Geometry check sheet. Reference: the model listing, model coordinates, mm. A direction names the side the tool comes from. Round coordinates to 2 decimals unless told otherwise and drop trailing zeros. Order: outer loops, then holes, each group sorted by start corner. A loop starts at its lowest first (then second) coordinate and runs counter-clockwise, first axis right, second up.
```python
from build123d import *

# Parameters (mm, degrees)
ESQUISSE1_W     = 40
ESQUISSE1_H     = 30
ESQUISSE1_R     = 2.5
BASE_DEPTH      = 10
EXT_R           = 5
ESQUISSE2_R     = 4
ACCES_VIS_DEPTH = 5


with BuildPart() as part:
    # Esquisse1 → BASE (new body)
    with BuildSketch(Plane(origin=(0, 0, 0), x_dir=(1, 0, 0), z_dir=(0, 1, 0))):
        Rectangle(ESQUISSE1_W, ESQUISSE1_H)
        with Locations(Location((0, 0, 0), (0, 0, 270))):
            Circle(ESQUISSE1_R, mode=Mode.SUBTRACT)
    extrude(amount=BASE_DEPTH)

    # EXT
    ext_edges = [part.edges().sort_by_distance(p)[0] for p in [
        (0, 0, -15),
        (20, 0, 0),
        (0, 0, 15),
        (-20, 0, 0),
    ]]
    fillet(ext_edges, radius=EXT_R)

    # Esquisse2 → ACCES VIS (cut)
    with BuildSketch(Plane(origin=(0, 0, 0), x_dir=(-1, 0, 0), z_dir=(0, -1, 0))):
        with Locations(Location((0, 0, 0), (0, 0, 90))):
            Circle(ESQUISSE2_R)
    extrude(amount=-ACCES_VIS_DEPTH, mode=Mode.SUBTRACT)


solid = part.part
```
(1) Sectioned sample at D-D, the plane z = -9. Record the cut outline in (x, y), and give its area (3 significant figures).
Returned:
outline: (-20, 5) arc R5 ccw to (-15, 0) - (15, 0) arc R5 ccw to (20, 5) - (20, 10) - (-20, 10) - close
area: 389 mm2
(2) Depth check by flat-ended pin: P1, Ø9, axis at x = -0.5, z = 1, coming from the -Y side; P2, Ø1, axis at x = -5.5, z = -11.5, coming from the -Y side. Enter the tip coordinate at first touch or a pass-through.
Returned:
P1: stops at y = 0
P2: stops at y = 0.1
(3) Set-up check for faces 5 (the flat face through (2, 5, -2)), 6 (the flat face through (0, 10, -4)): record each of +Z, -Z, +X, -X, +Y, -Y from which the full face is reachable in a straight line by a thin tool's end or side.
Returned:
face 5: -Y
face 6: +Z, -Z, +X, -X, +Y
(4) Sectioned sample at A-A, the plane z = 0. Record the cut outline in (x, y).
Returned:
outline: (-20, 5) arc R5 ccw to (-15, 0) - (-4, 0) - (-4, 5) - (-2.5, 5) - (-2.5, 10) - (-20, 10) - close; (2.5, 5) - (4, 5) - (4, 0) - (15, 0) arc R5 ccw to (20, 5) - (20, 10) - (2.5, 10) - close
(5) Sectioned sample at B-B, the plane x = 0. Record the cut outline in (y, z).
Returned:
outline: (0, -10) arc R5 ccw to (5, -15) - (10, -15) - (10, -2.5) - (5, -2.5) - (5, -4) - (0, -4) - close; (0, 4) - (5, 4) - (5, 2.5) - (10, 2.5) - (10, 15) - (5, 15) arc R5 ccw to (0, 10) - close
(6) Draft check along Z on faces 1 (the cylindrical face through (0, 2, 14)), 2 (the cylindrical face through (-3.905, 2.465, 0.867)), 3 (the flat face through (20, 7, 0)), 4 (the cylindrical face through (0, 2, -14)). Enter one of: released by +Z, released by -Z, zero draft, split by the parting line, or undercut.
Returned:
face 1: released by +Z
face 2: undercut
face 3: zero draft
face 4: released by -Z
(7) Material ranges on line 1 (Z direction, x = 0, y = 8); line 2 (X direction, y = 7.2, z = 0); line 3 (Z direction, x = -0.5, y = 5.25), recorded low to high.
Returned:
line 1: z = -15 to -2.5, 2.5 to 15
line 2: x = -20 to -2.5, 2.5 to 20
line 3: z = -15 to -2.45, 2.45 to 15
(8) Sectioned sample at C-C, the plane y = 1. Record the cut outline in (x, z), and give its area (3 significant figures).
Returned:
outline: (-18, -13) - (18, -13) - (18, 13) - (-18, 13) - close; hole circle Ø8 at (0, 0)
area: 886 mm2
